from build123d import *

# Parameters (mm, degrees)
SKETCH1_R           = 19.05
SKETCH1_R_2         = 15.875
BOSS_EXTRUDE1_DEPTH = 31.75
CUT_EXTRUDE2_DEPTH  = 32.75
CUT_EXTRUDE3_DEPTH  = 32.75


with BuildPart() as part:
    # Sketch1 → Boss-Extrude1 (new body)
    with BuildSketch(Plane(origin=(0, 0, 0), x_dir=(0, 0, -1), z_dir=(1, 0, 0))):
        Circle(SKETCH1_R)
        Circle(SKETCH1_R_2, mode=Mode.SUBTRACT)
    extrude(amount=BOSS_EXTRUDE1_DEPTH)

    # Sketch2 → Cut-Extrude2 (cut, through all)
    with BuildSketch(Plane(origin=(31.75, 0, 0), x_dir=(0, 0, -1), z_dir=(1, 0, 0))):
        with BuildLine():
            Line((-15.875, 0), (-19.05, 0))
            ThreePointArc((-19.05, 0), (-16.497783942, 9.525), (-9.525, 16.497783942))
            Line((-9.525, 16.497783942), (-7.9375, 13.748153285))
            ThreePointArc((-7.9375, 13.748153285), (-13.748153285, 7.9375), (-15.875, 0))
        make_face()
    extrude(amount=-CUT_EXTRUDE2_DEPTH, mode=Mode.SUBTRACT)

    # Sketch3 → Cut-Extrude3 (cut, through all)
    with BuildSketch(Plane(origin=(31.75, 0, 0), x_dir=(0, 0, -1), z_dir=(1, 0, 0))):
        with BuildLine():
            Line((-19.05, 0), (-15.875, 0))
            ThreePointArc((-15.875, 0), (-15.772137022, -1.804250192), (-15.464881102, -3.585118898))
            Line((-15.464881102, -3.585118898), (-19.05, 0))
        make_face()
    extrude(amount=-CUT_EXTRUDE3_DEPTH, mode=Mode.SUBTRACT)


solid = part.part
Verification items for the finished model (mm, model axes). A direction names the side the tool comes from. Round coordinates to 2 decimals unless told otherwise and drop trailing zeros. Write each loop counter-clockwise with the first axis right and the second up, starting at its lowest first coordinate (ties: lowest second). Pieces come first, ordered by that corner, then holes.
(1) Section check D-D (z = 11). Enter the section's corners in (x, y).
Returned:
outline: (0, -15.55) - (31.75, -15.55) - (31.75, -11.45) - (0, -11.45) - close
(2) Depth check by flat-ended pin: pin 1 Ø12 at (x, y) = (26, -10.5) entering from -Z; pin 2 Ø10 at (x, y) = (26.5, -2) entering from +Z; pin 3 Ø8 at (x, y) = (8, 6.5) entering from -Z; pin 4 Ø6 at (x, z) = (15.5, -13.5) entering from +Y. Enter the tip coordinate at first touch or a pass-through.
Returned:
pin 1: stops at z = -18.51
pin 2: stops at z = 19.05
pin 3: stops at z = -18.89
pin 4: stops at y = 15.9
(3) Mould release check, pull along Z, two halves, no side actions. Record for faces 1 (the flat face through (0, -10, -13)), 2 (the flat face through (16.1, 15.14, 8.74)), 3 (the cylindrical face through (15.65, -6.83, -14.33)): pulls with the +Z half, pulls with the -Z half, needs draft (parallel to the pull), parting line crosses it, or undercut.
Returned:
face 1: needs draft
face 2: pulls with the +Z half
face 3: undercut
(4) Section check A-A (z = 0). Enter the section's corners in (x, y) (3 decimals).
Returned:
outline: (0, -19.05) - (31.75, -19.05) - (31.75, -15.875) - (0, -15.875) - close; (0, 15.875) - (31.75, 15.875) - (31.75, 19.05) - (0, 19.05) - close
(5) Section check B-B (y = -7). Enter the section's corners in (x, z).
Returned:
outline: (0, -17.72) - (31.75, -17.72) - (31.75, -14.25) - (0, -14.25) - close; (0, 14.25) - (31.75, 14.25) - (31.75, 17.72) - (0, 17.72) - close
(6) Material ranges on line 1 (Y direction, x = 7.5, z = 0) (3 decimals); line 2 (Y direction, x = 18, z = -2); line 3 (Z direction, x = 27.5, y = -9), recorded low to high.
Returned:
line 1: y = -19.05 to -15.875, 15.875 to 19.05
line 2: y = -18.94 to -15.75, 15.75 to 18.94
line 3: z = -16.79 to -13.08, 13.08 to 16.79
(7) Access from +Z, -Z, +X, -X, +Y, -Y to the whole of each face (thin tool, end or side, straight path). Record for faces 4 (the flat face through (16.1, -1.82, 17.23)), 5 (the cylindrical face through (15.65, -10.12, -16.14)).
Returned:
face 4: +X, -X, +Y
face 5: +X, -X
